```python
from build123d import *

# Parameters (mm, degrees)
SKETCH1_R           = 28.575
SKETCH1_R_2         = 11
SKETCH1_R_3         = 3.302
BOSS_EXTRUDE1_DEPTH = 3.175
SKETCH1_4_R         = 11
BOSS_EXTRUDE2_DEPTH = 3.175
SKETCH1_5_R         = 11
BOSS_EXTRUDE3_DEPTH = 24.825


with BuildPart() as part:
    # Sketch1 → Boss-Extrude1 (new body)
    with BuildSketch(Plane(origin=(0, 0, 0), x_dir=(1, 0, 0), z_dir=(0, 1, 0))):
        Circle(SKETCH1_R)
        Circle(SKETCH1_R_2, mode=Mode.SUBTRACT)
        with Locations((21.548, 0)):
            Circle(SKETCH1_R_3, mode=Mode.SUBTRACT)
        with Locations((0, -21.548)):
            Circle(SKETCH1_R_3, mode=Mode.SUBTRACT)
        with Locations((-21.548, 0)):
            Circle(SKETCH1_R_3, mode=Mode.SUBTRACT)
        with Locations((0, 21.548)):
            Circle(SKETCH1_R_3, mode=Mode.SUBTRACT)
    extrude(amount=BOSS_EXTRUDE1_DEPTH)

    # Sketch1_4 → Boss-Extrude2 (add)
    with BuildSketch(Plane(origin=(0, 0, 0), x_dir=(1, 0, 0), z_dir=(0, 1, 0))):
        Circle(SKETCH1_4_R)
    extrude(amount=BOSS_EXTRUDE2_DEPTH)

    # Sketch1_5 → Boss-Extrude3 (add)
    with BuildSketch(Plane(origin=(0, 0, 0), x_dir=(1, 0, 0), z_dir=(0, 1, 0))):
        Circle(SKETCH1_5_R)
        with BuildLine():
            ThreePointArc((-5.414213562, -2.585786438), (-1.325654296, 5.851721173), (6, 0))
            ThreePointArc((6, 0), (3.200412581, -5.075170865), (-2.585786438, -5.414213562))
            Line((-2.585786438, -5.414213562), (-3.889087297, -6.717514421))
            Line((-3.889087297, -6.717514421), (-6.717514421, -3.889087297))
            Line((-6.717514421, -3.889087297), (-5.414213562, -2.585786438))
        make_face(mode=Mode.SUBTRACT)
    extrude(amount=-BOSS_EXTRUDE3_DEPTH)


solid = part.part
```
For this review, take the finished solid that the model builds, in its own axes (mm). A direction names the side the tool comes from. Give positions to 0.01 mm unless a question says otherwise; leave off trailing zeros. Order: outer loops, then holes, each group sorted by start corner. A loop starts at its lowest first (then second) coordinate and runs counter-clockwise, first axis right, second up.
1) Wall thickness on line 1 (X direction, y = 0.95, z = 0) (3 decimals); line 2 (Z direction, x = 0, y = -17.75): over which ranges is each line inside the solid? List them lowest first.
2) For faces 4 (the face through (0, 0, 12)), 5 (the face through (1.524, 1.565, -18.619)), list the 3-axis set-ups (+Z, -Z, +X, -X, +Y, -Y) from which the entire face can be reached by the end or side of a thin tool; tool diameter is ignored.
3) Insertion check: pin 1 (1.5 mm diameter, centred on x = -1, y = -12.5, fed in from +Z); pin 2 (4 mm diameter, centred on x = -3, z = 0, fed in from -Y); pin 3 (10 mm diameter, centred on x = 6, y = -5.5, fed in from -Z); pin 4 (5.5 mm diameter, centred on x = 21.548, z = 0, fed in from +Y). Each pin has a flat end and moves straight along its axis. Give the tip position at first contact, or say it passes through.
4) Take a section at B-B (y = -10.75). Give the boundary of the cut face in (x, z), then the cut area to 3 significant figures.
5) The part is to be moulded in two halves that separate along Z. For faces 1 (the face through (-2.38, -12.24, 10.74)), 2 (the face through (5, -24.825, 5)), 3 (the face through (0, 0, 0)), say which applies: released by +Z, released by -Z, zero draft, split by the parting line, or undercut.
6) Take a section at C-C (z = 20.5). Give the boundary of the cut face in (x, y) (3 decimals), then the cut area to 3 significant figures.
7) Take a section at A-A (x = 0). Give the boundary of the cut face in (y, z) (3 decimals).
8) Take a section at D-D (x = -22). Give the boundary of the cut face in (y, z) (3 decimals).
Derived:
1. line 1: x = -28.575 to -24.85, -18.246 to 18.246, 24.85 to 28.575
1. line 2: z = -11 to -6, 6 to 11
2. face 4: -Y
2. face 5: +Y, -Y
3. pin 1: stops at z = 11
3. pin 2: stops at y = 0
3. pin 3: stops at z = -10.95
3. pin 4: passes through
4. outline: circle Ø22 at (0, 0); hole (-6.72, 3.89) - (-5.41, 2.59) arc R6 ccw (long way) to (-2.59, 5.41) - (-3.89, 6.72) - close
4. area: 261 mm2
5. face 1: split by the parting line
5. face 2: zero draft
5. face 3: undercut
6. outline: (-19.907, 0) - (-3.131, 0) - (-3.131, 3.175) - (-19.907, 3.175) - close; (3.131, 0) - (19.907, 0) - (19.907, 3.175) - (3.131, 3.175) - close
6. area: 107 mm2
7. outline: (-24.825, -11) - (0, -11) - (0, -18.246) - (3.175, -18.246) - (3.175, 18.246) - (0, 18.246) - (0, 11) - (-24.825, 11) - (-24.825, 6) - (0, 6) - (0, -6) - (-24.825, -6) - close; (0, -28.575) - (3.175, -28.575) - (3.175, -24.85) - (0, -24.85) - close; (0, 24.85) - (3.175, 24.85) - (3.175, 28.575) - (0, 28.575) - close
8. outline: (0, -18.235) - (3.175, -18.235) - (3.175, -3.271) - (0, -3.271) - close; (0, 3.271) - (3.175, 3.271) - (3.175, 18.235) - (0, 18.235) - close
